Work out the finished part from the listing and answer in its coordinate system (mm). A direction names the side the tool comes from. Coordinates: 2 decimals unless noted, no trailing zeros. Order: outer loops, then holes, each group sorted by start corner. A loop starts at its lowest first (then second) coordinate and runs counter-clockwise, first axis right, second up. Notation, with made-up numbers: M -11.75,-7 L 42.25,-7 A12 cw 42.25,1 Z; hole C 76.5,2.25 d9. An arc over 180 degrees is marked long. Use a Markdown table: item, result.
from build123d import *

# Parameters (mm, degrees)
SKETCH1_W          = 50
SKETCH1_H          = 50
SKETCH1_R          = 2
BODY_DEPTH         = 11.8
FILLET1_R          = 5
SKETCH2_R          = 3.05
C_BORES_DEPTH      = 1.5
CUT_EXTRUDE1_DEPTH = 9


with BuildPart() as part:
    # Sketch1 → Body (new body)
    with BuildSketch(Plane(origin=(0, 0, 0), x_dir=(0, 0, -1), z_dir=(1, 0, 0))):
        Rectangle(SKETCH1_W, SKETCH1_H)
        with Locations((-20, -20)):
            Circle(SKETCH1_R, mode=Mode.SUBTRACT)
        with Locations((-20, 20)):
            Circle(SKETCH1_R, mode=Mode.SUBTRACT)
        with Locations((20, 20)):
            Circle(SKETCH1_R, mode=Mode.SUBTRACT)
        with Locations((20, -20)):
            Circle(SKETCH1_R, mode=Mode.SUBTRACT)
    extrude(amount=BODY_DEPTH)

    # Fillet1
    fillet1_edges = [part.edges().sort_by_distance(p)[0] for p in [
        (5.9, -25, -25),
        (5.9, -25, 25),
        (5.9, 25, 25),
        (5.9, 25, -25),
    ]]
    fillet(fillet1_edges, radius=FILLET1_R)

    # Sketch2 → C'Bores (cut)
    with BuildSketch(Plane.ZY):
        with Locations((-20, -20)):
            Circle(SKETCH2_R)
        with Locations((-20, 20)):
            Circle(SKETCH2_R)
        with Locations((20, 20)):
            Circle(SKETCH2_R)
        with Locations((20, -20)):
            Circle(SKETCH2_R)
    extrude(amount=-C_BORES_DEPTH, mode=Mode.SUBTRACT)

    # Sketch3 → Cut-Extrude1 (cut)
    with BuildSketch(Plane.ZY):
        with BuildLine():
            Line((-25, -19.625988463), (-20.087724144, -14.713712607))
            ThreePointArc((-20.087724144, -14.713712607), (-24.9, 0), (-20.087724144, 14.713712607))
            Line((-20.087724144, 14.713712607), (-25, 19.625988463))
            Line((-25, 19.625988463), (-25, -19.625988463))
        make_face()
        with BuildLine():
            Line((-19.625988463, -25), (-14.713712607, -20.087724144))
            ThreePointArc((-14.713712607, -20.087724144), (0, -24.9), (14.713712607, -20.087724144))
            Line((14.713712607, -20.087724144), (19.625988463, -25))
            Line((19.625988463, -25), (-19.625988463, -25))
        make_face()
        with BuildLine():
            Line((-19.625988463, 25), (-14.713712607, 20.087724144))
            ThreePointArc((-14.713712607, 20.087724144), (0, 24.9), (14.713712607, 20.087724144))
            Line((14.713712607, 20.087724144), (19.625988463, 25))
            Line((19.625988463, 25), (-19.625988463, 25))
        make_face()
        with BuildLine():
            Line((25, 19.625988463), (20.087724144, 14.713712607))
            ThreePointArc((20.087724144, 14.713712607), (24.9, 0), (20.087724144, -14.713712607))
            Line((20.087724144, -14.713712607), (25, -19.625988463))
            Line((25, -19.625988463), (25, 19.625988463))
        make_face()
    extrude(amount=-CUT_EXTRUDE1_DEPTH, mode=Mode.SUBTRACT)


solid = part.part
1. Section D-D on x = 5.25 is taken. Determine the outline of the cut face in (y, z), then the cut area to 3 significant figures.
Answers below:
| item | result |
|---|---|
| outline | M -25,-20 A5 ccw -20,-25 L -19.63,-25 L -14.71,-20.09 A24.9 ccw 14.71,-20.09 L 19.63,-25 L 20,-25 A5 ccw 25,-20 L 25,-19.63 L 20.09,-14.71 A24.9 ccw 20.09,14.71 L 25,19.63 L 25,20 A5 ccw 20,25 L 19.63,25 L 14.71,20.09 A24.9 ccw -14.71,20.09 L -19.63,25 L -20,25 A5 ccw -25,20 L -25,19.63 L -20.09,14.71 A24.9 ccw -20.09,-14.71 L -25,-19.63 Z; hole C -20,-20 d4; hole C -20,20 d4; hole C 20,-20 d4; hole C 20,20 d4 |
| area | 2,140 mm² |
2. For a pull along Y with two mould halves and no side action, classify faces 6 (the face through (7, -18, -20)), 7 (the face through (4.437, 22.578, -17.204)), 8 (the face through (9, 24.8, 4.1)) as +Y half, -Y half, draft (parallel to the pull), parting line (faces both ways), or undercut.
Answers below:
| item | result |
|---|---|
| face 6 | undercut |
| face 7 | +Y half |
| face 8 | draft |
3. For faces 1 (the face through (0.74, -17.43, 21.64)), 2 (the face through (4.437, 17.135, -22.509)), 3 (the face through (4.437, -22.578, -17.204)), 4 (the face through (7, 22, -20)), 5 (the face through (4.4, 0.2, 24.9)), determine the directions among +Z, -Z, +X, -X, +Y, -Y from which every point of the face is accessible in a straight line to the end or side of a thin tool.
Answers below:
| item | result |
|---|---|
| face 1 | -X |
| face 2 | -Z, -X |
| face 3 | -X, -Y |
| face 4 | +X, -X |
| face 5 | +Z, -X |
4. Find the intervals of material crossed by probe 1 along Y at (x, z) = (4.5, 20); probe 2 along Y at (x, z) = (1.2, -20), in increasing order.
Answers below:
| item | result |
|---|---|
| probe 1 | -25 to -22, -18 to 18, 22 to 25 |
| probe 2 | -25 to -23.05, -16.95 to 16.95, 23.05 to 25 |
5. Section C-C on z = 13.5 is taken. Determine the outline of the cut face in (x, y), then the cut area to 3 significant figures.
Answers below:
| item | result |
|---|---|
| outline | M 0,-20.92 L 9,-20.92 L 9,-25 L 11.8,-25 L 11.8,25 L 9,25 L 9,20.92 L 0,20.92 Z |
| area | 517 mm² |
6. Section B-B on y = 7 is taken. Determine the outline of the cut face in (x, z), then the cut area to 3 significant figures.
Answers below:
| item | result |
|---|---|
| outline | M 0,-23.9 L 9,-23.9 L 9,-25 L 11.8,-25 L 11.8,25 L 9,25 L 9,23.9 L 0,23.9 Z |
| area | 570 mm² |
7. Flat-ended cylindrical pins translate along their axes: P1, Ø1.8, axis at y = -18.5, z = 20.5, coming from the -X side; P2, Ø1, axis at x = 6.5, y = -10.5, coming from the -Z side; P3, Ø3.5, axis at y = -20, z = -20, coming from the -X side; P4, Ø2, axis at x = 5.5, z = 2, coming from the +Y side. Find the tip coordinate at first contact, or state that the pin passes through.
Answers below:
| item | result |
|---|---|
| P1 | x = 1.5 |
| P2 | z = -22.8 |
| P3 | through |
| P4 | y = 24.88 |
8. Section A-A on x = 10.5 is taken. Determine the outline of the cut face in (y, z).
Answers below:
| item | result |
|---|---|
| outline | M -25,-20 A5 ccw -20,-25 L 20,-25 A5 ccw 25,-20 L 25,20 A5 ccw 20,25 L -20,25 A5 ccw -25,20 Z; hole C -20,-20 d4; hole C -20,20 d4; hole C 20,-20 d4; hole C 20,20 d4 |
